```python
from build123d import *

# Parameters (mm, degrees)
F1_DEPTH = 2.54


with BuildPart() as f1:
    # F0 (on Front) → F1 (new body)
    with BuildSketch(Plane.XZ):
        Polygon((-9.525, 6.35), (-9.525, -6.35), (-4.445, -6.35), (-9.067422, -19.05), (-6.527422, -19.05), (-4.216211, -12.7), (4.216211, -12.7), (6.527422, -19.05), (9.067422, -19.05), (4.445, -6.35), (9.525, -6.35), (9.525, 6.35), align=None)
        Polygon((-1.905, -6.35), (1.905, -6.35), (3.291727, -10.16), (-3.291727, -10.16), align=None, mode=Mode.SUBTRACT)
    extrude(amount=F1_DEPTH)

    # F4 (on offset) → F5 section 0
    with BuildSketch(Plane.XZ.offset(-3.81)):
        Polygon((-5.912923, -17.383784), (-8.452923, -17.383784), (-8.887289, -18.577194), (-6.347289, -18.577194), align=None)
    # F2 (on face) → F5 section 1
    with BuildSketch(Plane(origin=(0, 0, 0), x_dir=(-1, 0, 0), z_dir=(0, 1, 0))):
        Polygon((8.633056, -17.85659), (6.093056, -17.85659), (6.527422, -19.05), (9.067422, -19.05), align=None)
    loft()

    # F4 (on offset) → F6 section 0
    with BuildSketch(Plane.XZ.offset(-3.81)):
        Polygon((8.887289, -18.577194), (8.452923, -17.383784), (5.912923, -17.383784), (6.347289, -18.577194), align=None)
    # F2 (on face) → F6 section 1
    with BuildSketch(Plane(origin=(0, 0, 0), x_dir=(-1, 0, 0), z_dir=(0, 1, 0))):
        Polygon((-8.633056, -17.85659), (-9.067422, -19.05), (-6.527422, -19.05), (-6.093056, -17.85659), align=None)
    loft()


solid = f1.part
```
Source: CAD feature listing. Evaluate the final solid. Frame: model axes, mm. A direction names the side the tool comes from. Coordinates: 2 decimals unless noted, no trailing zeros. Write each loop counter-clockwise with the first axis right and the second up, starting at its lowest first coordinate (ties: lowest second). Pieces come first, ordered by that corner, then holes. Notation, with made-up numbers: (4, 56) - (42, 56) arc R10 cw to (42, 66) - close; hole circle Ø8 at (-18, 17.5). An arc over 180 degrees is marked (long way). Answer as a JSON object with one key per item and string values.
Q1. Set-up query: faces 1 (the flat face through (0, -1, -6.35)), 2 (the flat face through (6.79, -1.25, -12.79)). Return all of +Z, -Z, +X, -X, +Y, -Y with unobstructed straight access to the full face (end or side cutting, diameter ignored); none if empty.
Ans:
{"face 1": "+Y, -Y", "face 2": "+X, +Y, -Y"}
Q2. First-contact query: pin 1 Ø1.5 at (y, z) = (2, 0) entering from -X; pin 2 Ø2 at (x, y) = (-0.5, -1) entering from -Z; pin 3 Ø9.5 at (x, z) = (4, -4.5) entering from +Y; pin 4 Ø1.5 at (x, y) = (6, 1.5) entering from -Z (3 decimals). Flat tips, straight axial feed; report the tip coordinate or a pass-through.
Ans:
{"pin 1": "passes through", "pin 2": "stops at z = -12.7", "pin 3": "stops at y = 0", "pin 4": "stops at z = -18.935"}
Q3. Section query D-D, the plane z = 4. Output: boundary loops of the cut face in (x, y) (3 decimals).
Ans:
{"outline": "(-9.525, -2.54) - (9.525, -2.54) - (9.525, 0) - (-9.525, 0) - close"}
Q4. Section query B-B, the plane x = -1.5. Output: boundary loops of the cut face in (y, z), plus the area to 3 significant figures.
Ans:
{"outline": "(-2.54, -12.7) - (0, -12.7) - (0, -10.16) - (-2.54, -10.16) - close; (-2.54, -6.35) - (0, -6.35) - (0, 6.35) - (-2.54, 6.35) - close", "area": "38.7 mm2"}
Q5. Material intervals for line 1 (Z direction, x = 0.25, y = -1.5); line 2 (Y direction, x = 8, z = -1.5); line 3 (Z direction, x = 7, y = 0.5), sorted ascending. Write a range as [from, to].
Ans:
{"line 1": "z = [-12.7, -10.16], [-6.35, 6.35]", "line 2": "y = [-2.54, 0]", "line 3": "z = [-18.99, -17.79]"}
Q6. Section query A-A, the plane y = -1.75. Output: boundary loops of the cut face in (x, z) (3 decimals).
Ans:
{"outline": "(-9.525, -6.35) - (-4.445, -6.35) - (-9.067, -19.05) - (-6.527, -19.05) - (-4.216, -12.7) - (4.216, -12.7) - (6.527, -19.05) - (9.067, -19.05) - (4.445, -6.35) - (9.525, -6.35) - (9.525, 6.35) - (-9.525, 6.35) - close; hole (-3.292, -10.16) - (3.292, -10.16) - (1.905, -6.35) - (-1.905, -6.35) - close"}
Q7. Draft query along Z for faces 3 (the flat face through (0, -1, 6.35)), 4 (the flat face through (-7, 3.81, -18)), 5 (the flat face through (0, -1, -12.7)), 6 (the flat face through (7, -1, -6.35)). Return one class per face: released by +Z, released by -Z, zero draft, split by the parting line, or undercut.
Ans:
{"face 3": "released by +Z", "face 4": "zero draft", "face 5": "released by -Z", "face 6": "undercut"}
Q8. Section query C-C, the plane z = -9.5. Output: boundary loops of the cut face in (x, y).
Ans:
{"outline": "(-5.59, -2.54) - (-3.05, -2.54) - (-3.05, 0) - (-5.59, 0) - close; (3.05, -2.54) - (5.59, -2.54) - (5.59, 0) - (3.05, 0) - close"}
